Geometry: final body of the model. Coordinates: model frame, mm. A direction names the side the tool comes from. Round coordinates to 2 decimals unless told otherwise and drop trailing zeros. Order: outer loops, then holes, each group sorted by start corner. A loop starts at its lowest first (then second) coordinate and runs counter-clockwise, first axis right, second up. Notation, with made-up numbers: (-8, -18) - (11, -18) arc R12 ccw to (11, -3) - close; hole circle Ø1 at (38.25, -31.75). An arc over 180 degrees is marked (long way). Put each result on its own line as item: value. Start each with the question number.
(1) Section B-B (x = -42.5). Output: boundary loops of the cut face in (y, z), and give its area (3 significant figures).
(2) Section C-C (z = -14.25). Output: boundary loops of the cut face in (x, y), and give its area (3 significant figures).
(3) Pin query (flat end, axial travel): P1, Ø5, axis at y = 2, z = -15.5, coming from the -X side; P2, Ø5, axis at y = 7.5, z = -5, coming from the +X side; P3, Ø8, axis at x = 42.5, y = -14, coming from the -Z side. Return the tip coordinate at first contact, or that it passes through.
(4) Access query for faces 1 (the face through (-60, -17, -10)), 2 (the face through (60, -17, -10)), 3 (the face through (-1, 1, -20)). Directions: +Z, -Z, +X, -X, +Y, -Y. A direction counts if a zero-diameter tool reaches every point of the face in a straight line with its end or side. Return the directions, or none.
(5) Section A-A (y = -14). Output: boundary loops of the cut face in (x, z).
(6) Material intervals for L1, parallel to Y at x = 42.5, z = -10.5; L2, parallel to X at y = -26.5, z = -2.5; L3, parallel to X at y = 14, z = -11.5, sorted ascending. Write a range as [from, to].
(7) Section D-D (x = 57.5). Output: boundary loops of the cut face in (y, z).
(8) Pull-direction query (X, two-part tool) for faces 4 (the face through (-82.5, 41, -10)), 5 (the face through (36, -14, -10)), 6 (the face through (82.5, 41, -10)), 7 (the face through (-49, -14, -10)); classes: released by +X, released by -X, zero draft, split by the parting line, or undercut.
Solid Edge part; units mm, degrees
sketch "Sketch1" plane through (0, 0, 0) normal (0, 0, 1) x (1, 0, 0)
  line L0 (-82.5, -42.5) -> (82.5, -42.5)
  line L1 (82.5, -42.5) -> (82.5, 42.5)
  line L2 (82.5, 42.5) -> (-82.5, 42.5)
  line L3 (-82.5, 42.5) -> (-82.5, -42.5)
extrude "Protrusion1" add sketch "Sketch1" against normal blind 20
sketch "Sketch2" plane through (0, 0, 0) normal (0, 0, 1) x (1, 0, 0)
  circle A0 centre (-42.5, -14) radius 6.5
  circle A1 centre (-117.5, -7) radius 57.5
extrude "ExtrudedCutout_1" cut sketch "Sketch2" against normal blind 20
sketch "Sketch3" plane through (0, 0, 0) normal (0, 0, 1) x (1, 0, 0)
  circle A0 centre (117.5, -7) radius 57.5
  circle A1 centre (42.5, -14) radius 6.5
extrude "ExtrudedCutout_2" cut sketch "Sketch3" against normal blind 20
sketch "Sketch4" plane through (0, 0, 0) normal (0, 0, 1) x (1, 0, 0)
  line L0 (60, -7) -> (82.5, -7)
  line L1 (82.5, -7) -> (82.5, -50.0706)
  line L2 (82.5, -50.0706) -> (60, -50.0706)
  line L3 (60, -50.0706) -> (60, -7)
  line L4 (-60, -7) -> (-88.75, -7)
  line L5 (-88.75, -7) -> (-88.75, -50.6186)
  line L6 (-88.75, -50.6186) -> (-60, -50.6186)
  line L7 (-60, -50.6186) -> (-60, -7)
extrude "ExtrudedCutout_3" cut sketch "Sketch4" against normal blind 20
fillet "Round_2" radius 15 2 edges at (60, -42.5, -10) (-60, -42.5, -10)
Checks:
1. outline: (-42.5, -20) - (-20.5, -20) - (-20.5, 0) - (-42.5, 0) - close; (-7.5, -20) - (42.5, -20) - (42.5, 0) - (-7.5, 0) - close
1. area: 1,440 mm²
2. outline: (-82.5, 38.62) arc R57.5 cw to (-60, -7) - (-60, -27.5) arc R15 ccw to (-45, -42.5) - (45, -42.5) arc R15 ccw to (60, -27.5) - (60, -7) arc R57.5 cw to (82.5, 38.62) - (82.5, 42.5) - (-82.5, 42.5) - close; hole circle Ø13 at (-42.5, -14); hole circle Ø13 at (42.5, -14)
2. area: 10,600 mm²
3. P1: stops at x = -61.16
3. P2: stops at x = 62.57
3. P3: passes through
4. face 1: +Z, -Z, -X, -Y
4. face 2: +Z, -Z, +X, -Y
4. face 3: -Z, +X, -X, +Y, -Y
5. outline: (-60, -20) - (-49, -20) - (-49, 0) - (-60, 0) - close; (-36, -20) - (36, -20) - (36, 0) - (-36, 0) - close; (49, -20) - (60, -20) - (60, 0) - (49, 0) - close
6. L1: y = [-42.5, -20.5], [-7.5, 42.5]
6. L2: x = [-60, 60]
6. L3: x = [-63.97, 63.97]
7. outline: (-35.79, -20) - (42.5, -20) - (42.5, 0) - (-35.79, 0) - close
8. face 4: released by -X
8. face 5: undercut
8. face 6: released by +X
8. face 7: undercut
